The model under review builds one solid part; all positions refer to its coordinate system, in mm. Give positions to 0.01 mm unless a question says otherwise; leave off trailing zeros. Order: outer loops, then holes, each group sorted by start corner. A loop starts at its lowest first (then second) coordinate and runs counter-clockwise, first axis right, second up.
```python
from build123d import *

# Parameters (mm, degrees)
F0_W     = 75
F0_H     = 7
F1_DEPTH = 3.5
F2_W     = 68
F2_H     = 3
F3_DEPTH = 1.5
F4_R     = 1


with BuildPart() as f1:
    # F0 (on Top) → F1 (new body)
    with BuildSketch(Plane.XY):
        Rectangle(F0_W, F0_H)
    extrude(amount=F1_DEPTH)

    # F2 (on face) → F3 (cut)
    with BuildSketch(Plane.XY.offset(3.5)):
        with Locations((0, 0.834541)):
            Rectangle(F2_W, F2_H)
    extrude(amount=-F3_DEPTH, mode=Mode.SUBTRACT)

    # F4
    f4_edges = [f1.edges().sort_by_distance(p)[0] for p in [
        (0, -3.5, 0),
        (37.5, 0, 0),
        (0, 3.5, 0),
        (-37.5, 0, 0),
    ]]
    fillet(f4_edges, radius=F4_R)


solid = f1.part
```
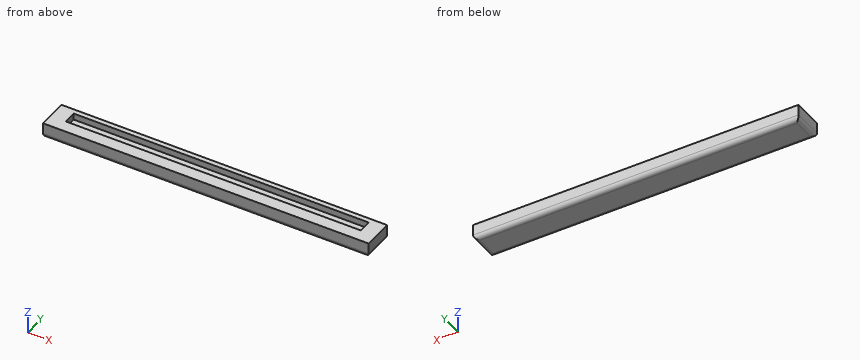
1. Take a section at C-C (y = 0). Write out the cut boundary in (x, z).
2. To check wall thickness, follow line 1 (X direction, y = 2.25, z = 3.2); line 2 (Z direction, x = 9.5, y = 1); line 3 (Y direction, x = -12.5, z = 3.25). State the ranges of each line that lie inside material, in increasing order.
3. Take a section at B-B (x = -24). Write out the cut boundary in (y, z).
4. Take a section at A-A (z = 2.75). Write out the cut boundary in (x, y), and give its area (3 significant figures).
5. Insertion check: pin 1 (0.9 mm diameter, centred on x = -10.5, y = 0.5, fed in from +Z). The pin has a flat end and moves straight along its axis. Give the tip position at first contact, or say it passes through.
Answer:
1. outline: (-37.5, 1) arc R1 ccw to (-36.5, 0) - (36.5, 0) arc R1 ccw to (37.5, 1) - (37.5, 3.5) - (34, 3.5) - (34, 2) - (-34, 2) - (-34, 3.5) - (-37.5, 3.5) - close
2. line 1: x = -37.5 to -34, 34 to 37.5
2. line 2: z = 0 to 2
2. line 3: y = -3.5 to -0.67, 2.33 to 3.5
3. outline: (-3.5, 1) arc R1 ccw to (-2.5, 0) - (2.5, 0) arc R1 ccw to (3.5, 1) - (3.5, 3.5) - (2.33, 3.5) - (2.33, 2) - (-0.67, 2) - (-0.67, 3.5) - (-3.5, 3.5) - close
4. outline: (-37.5, -3.5) - (37.5, -3.5) - (37.5, 3.5) - (-37.5, 3.5) - close; hole (-34, -0.67) - (34, -0.67) - (34, 2.33) - (-34, 2.33) - close
4. area: 321 mm2
5. pin 1: stops at z = 2
